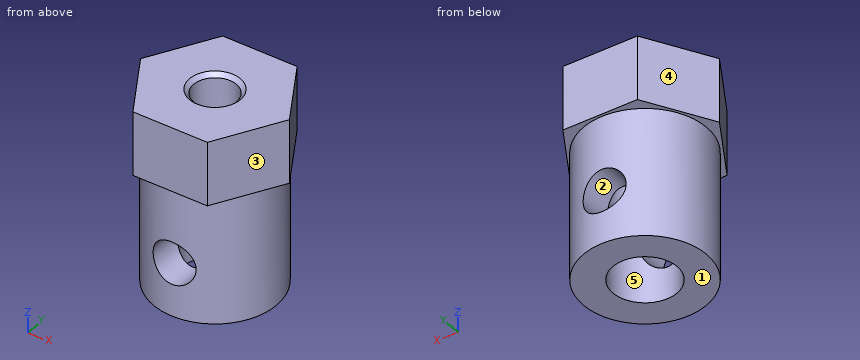
```python
from build123d import *

# Parameters (mm, degrees)
EXTRUDE_1_DEPTH              = 6
SKETCH_2_W                   = 5.75
SKETCH_2_H                   = 12
HOLE_WIZARD_M4_1_D           = 4
HOLE_WIZARD_M4_1_CBORE_D     = 6
HOLE_WIZARD_M4_1_CBORE_DEPTH = 12
SKETCH_7_R                   = 2
CUT_EXTRUDE_1_DEPTH          = 19.167622299
CHAMFER_1_SIZE               = 0.375


with BuildPart() as part:
    # 草图1 → 凸台-拉伸1 (new body)
    with BuildSketch(Plane.XY.offset(6)):
        Polygon((-3.464101615, -6), (3.464101615, -6), (6.92820323, 0), (3.464101615, 6), (-3.464101615, 6), (-6.92820323, 0), align=None)
    extrude(amount=-EXTRUDE_1_DEPTH)

    # 草图2 → 旋转1 (revolve)
    with BuildSketch(Plane(origin=(0, 0, 0), x_dir=(1, 0, 0), z_dir=(0, 1, 0))):
        with Locations((2.875, 6)):
            Rectangle(SKETCH_2_W, SKETCH_2_H)
    revolve(axis=Axis((0, 0, -12), (0, 0, 1)))

    # M4 六角头机械螺钉的柱形沉头孔1 (through all)
    with Locations(Plane(origin=(0, 0, -12), x_dir=(-1, 0, 0), z_dir=(0, 0, -1))):
        with Locations((0, 0)):
            CounterBoreHole(HOLE_WIZARD_M4_1_D / 2, HOLE_WIZARD_M4_1_CBORE_D / 2, HOLE_WIZARD_M4_1_CBORE_DEPTH)

    # 草图7 → 切除-拉伸1 (cut, through all)
    with BuildSketch(Plane(origin=(0, 5.75, 0), x_dir=(1, 0, 0), z_dir=(0, 1, 0))):
        with Locations(Location((0, 7, 0), (0, 0, 270))):
            Circle(SKETCH_7_R)
    extrude(amount=-CUT_EXTRUDE_1_DEPTH, mode=Mode.SUBTRACT)

    # 倒角1
    chamfer_1_edges = [part.edges().sort_by_distance(p)[0] for p in [
        (-2, 0, 6),
    ]]
    chamfer(chamfer_1_edges, length=CHAMFER_1_SIZE)


solid = part.part
```
Input: part model. Units: mm. Frame: model coordinates. Face numbers are marked on the shaded views. A direction names the side the tool comes from. Give positions to 0.01 mm unless a question says otherwise; leave off trailing zeros. Order: outer loops, then holes, each group sorted by start corner. A loop starts at its lowest first (then second) coordinate and runs counter-clockwise, first axis right, second up. Notation, with made-up numbers: (29.25, -32.5) - (59.25, -32.5) arc R32 cw to (59.25, -0.5) - close; hole circle Ø8 at (81, 22). An arc over 180 degrees is marked (long way). One line per item, written item: value.
1. Cut plane C-C, the plane z = -6.25. Output: boundary loops of the cut face in (x, y).
Determined:
outline: (-1.85, -5.44) - (-1.85, -2.36) arc R3 cw to (-1.85, 2.36) - (-1.85, 5.44) arc R5.75 ccw to start; (1.85, -5.44) arc R5.75 ccw to (1.85, 5.44) - (1.85, 2.36) arc R3 cw to (1.85, -2.36) - close
2. Reachability of the marked faces 4 and 5 from +Z, -Z, +X, -X, +Y, -Y: full face, straight path, thin tool, end or side. Return the list, or none.
Determined:
face 4: +Z, -Z, -X, +Y
face 5: -Z
3. Pin query (flat end, axial travel): pin 1 Ø3.5 at (x, z) = (0, -7) entering from -Y; pin 2 Ø3 at (y, z) = (-2, 2) entering from -X; pin 3 Ø2 at (x, y) = (-2, -1) entering from -Z; pin 4 Ø1.5 at (y, z) = (3.5, -6) entering from +X. Return the tip coordinate at first contact, or that it passes through.
Determined:
pin 1: through
pin 2: x = -6.64
pin 3: z = -12
pin 4: x = 5.05
4. Cut plane D-D, the plane y = 5. Output: boundary loops of the cut face in (x, z).
Determined:
outline: (-4.04, 0) - (-2.84, 0) - (-2.84, -12) - (2.84, -12) - (2.84, 0) - (4.04, 0) - (4.04, 6) - (-4.04, 6) - close; hole circle Ø4 at (0, -7)
5. Line query: probe 1 along Z at (x, y) = (0, -4.7); probe 2 along Y at (x, z) = (0, -3.75); probe 3 along X at (y, z) = (3.1, -7). Output: solid intervals per line, ascending.
Determined:
probe 1: -12 to -9, -5 to 6
probe 2: -5.75 to -3, 3 to 5.75
probe 3: -4.84 to -2, 2 to 4.84
6. Draft query along X for the marked faces 1, 2 and 3. Return one class per face: released by +X, released by -X, zero draft, split by the parting line, or undercut.
Determined:
face 1: zero draft
face 2: undercut
face 3: released by +X
7. Cut plane A-A, the plane x = 0. Output: boundary loops of the cut face in (y, z) (3 decimals), and give its area (3 significant figures).
Determined:
outline: (-6, 0) - (-5.75, 0) - (-5.75, -5) - (-3, -5) - (-3, 0) - (-2, 0) - (-2, 5.625) - (-2.375, 6) - (-6, 6) - close; (-5.75, -12) - (-3, -12) - (-3, -9) - (-5.75, -9) - close; (2, 0) - (3, 0) - (3, -5) - (5.75, -5) - (5.75, 0) - (6, 0) - (6, 6) - (2.375, 6) - (2, 5.625) - close; (3, -12) - (5.75, -12) - (5.75, -9) - (3, -9) - close
area: 91.9 mm2
8. Cut plane B-B, the plane z = 4.25. Output: boundary loops of the cut face in (x, y), and give its area (3 significant figures).
Determined:
outline: (-6.93, 0) - (-3.46, -6) - (3.46, -6) - (6.93, 0) - (3.46, 6) - (-3.46, 6) - close; hole circle Ø4 at (0, 0)
area: 112 mm2
